Here's how the part is built. I have some questions about the finished solid (model axes, mm). Coordinates: 2 decimals unless noted, no trailing zeros. Write each loop counter-clockwise with the first axis right and the second up, starting at its lowest first coordinate (ties: lowest second). Pieces come first, ordered by that corner, then holes. Notation, with made-up numbers: (-8.75, 26.5) -> (41.25, 26.5) arc R31 cw to (41.25, 55.5) -> close; hole circle Ø1 at (46.25, -15.75). An arc over 180 degrees is marked (long way). Put each result on its own line as item: value.
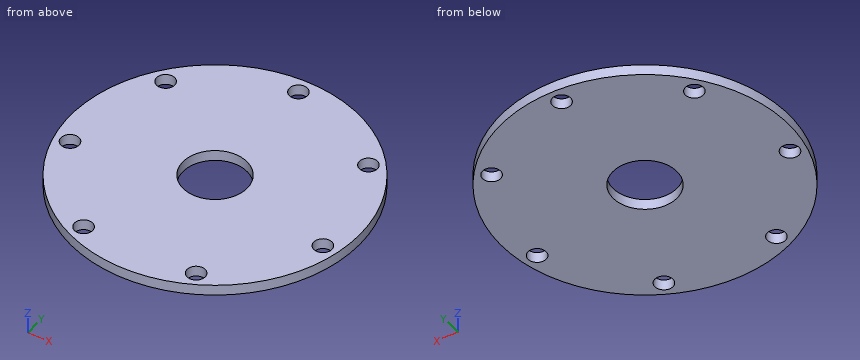
```python
from build123d import *

# Parameters (mm, degrees)
ESQUISSE1_R        = 67.5
ESQUISSE1_R_2      = 4.25
ESQUISSE1_R_3      = 15
BOSS_EXTRU_1_DEPTH = 5


with BuildPart() as part:
    # Esquisse1 → Boss.-Extru.1 (new body)
    with BuildSketch(Plane.XY):
        Circle(ESQUISSE1_R)
        with Locations((0, 60.5)):
            Circle(ESQUISSE1_R_2, mode=Mode.SUBTRACT)
        with Locations((47.300804689, 37.721133012)):
            Circle(ESQUISSE1_R_2, mode=Mode.SUBTRACT)
        with Locations((58.983138687, -13.462516504)):
            Circle(ESQUISSE1_R_2, mode=Mode.SUBTRACT)
        with Locations((26.249966217, -54.508616508)):
            Circle(ESQUISSE1_R_2, mode=Mode.SUBTRACT)
        with Locations((-26.249966217, -54.508616508)):
            Circle(ESQUISSE1_R_2, mode=Mode.SUBTRACT)
        with Locations((-58.983138687, -13.462516504)):
            Circle(ESQUISSE1_R_2, mode=Mode.SUBTRACT)
        with Locations((-47.300804689, 37.721133012)):
            Circle(ESQUISSE1_R_2, mode=Mode.SUBTRACT)
        Circle(ESQUISSE1_R_3, mode=Mode.SUBTRACT)
    extrude(amount=BOSS_EXTRU_1_DEPTH)


solid = part.part
```
Item 1: Please list where these lines run through material, in increasing order: line 1 along X through (y, z) = (-10, 1.45); line 2 along X through (y, z) = (36.5, 4.75); line 3 along X through (y, z) = (-13.5, 4.05). Write a range as from..to.
Output:
line 1: x = -66.76..-61.45, -56.52..-11.18, 11.18..56.52, 61.45..66.76
line 2: x = -56.78..-51.37, -43.23..43.23, 51.37..56.78
line 3: x = -66.14..-63.23, -54.73..-6.54, 6.54..54.73, 63.23..66.14
Item 2: Imagine slicing it at D-D on z = 2.8. State how many separate pieces and enclosed holes the cut face has, then the cut area to 3 significant figures.
Output:
separate pieces: 1
enclosed holes: 8
area: 13,200 mm²
Item 3: For P1, Ø3, axis at y = 18.5, z = 2.5, coming from the +X side; P2, Ø2, axis at y = 5, z = 2.5, coming from the -X side; P3, Ø2, axis at x = -40.5, z = 1, coming from the +Y side, each with a flat end and sliding along its axis, tell me the tip position at first contact or that it passes through.
Output:
P1: stops at x = 65.32
P2: stops at x = -67.38
P3: stops at y = 54.74
Item 4: Imagine slicing it at C-C on x = -25. Write out the boundary of the cut face in (y, z), then the cut area to 3 significant figures.
Output:
outline: (-62.7, 0) -> (-58.57, 0) -> (-58.57, 5) -> (-62.7, 5) -> close; (-50.45, 0) -> (62.7, 0) -> (62.7, 5) -> (-50.45, 5) -> close
area: 586 mm²
Item 5: Imagine slicing it at B-B on x = 0. Write out the boundary of the cut face in (y, z).
Output:
outline: (-67.5, 0) -> (-15, 0) -> (-15, 5) -> (-67.5, 5) -> close; (15, 0) -> (56.25, 0) -> (56.25, 5) -> (15, 5) -> close; (64.75, 0) -> (67.5, 0) -> (67.5, 5) -> (64.75, 5) -> close
Item 6: Imagine slicing it at A-A on y = 0. Write out the boundary of the cut face in (x, z), then the cut area to 3 significant figures.
Output:
outline: (-67.5, 0) -> (-15, 0) -> (-15, 5) -> (-67.5, 5) -> close; (15, 0) -> (67.5, 0) -> (67.5, 5) -> (15, 5) -> close
area: 525 mm²
